Answer from the drawing. Dimensions are ordinates in mm from the lowest x, y and z of the part. Give positions to 0.01 mm unless a question says otherwise; leave off trailing zeros. Order: outer loops, then holes, each group sorted by start corner. A loop starts at its lowest first (then second) coordinate and runs counter-clockwise, first axis right, second up. Notation, with made-up numbers: (-28, 17) - (7, 17) arc R28 cw to (7, 50) - close; hole circle Ø7 at (83.25, -30.5). An arc over 180 degrees is marked (long way). Write each question's results on one line, items separated by ' | '.
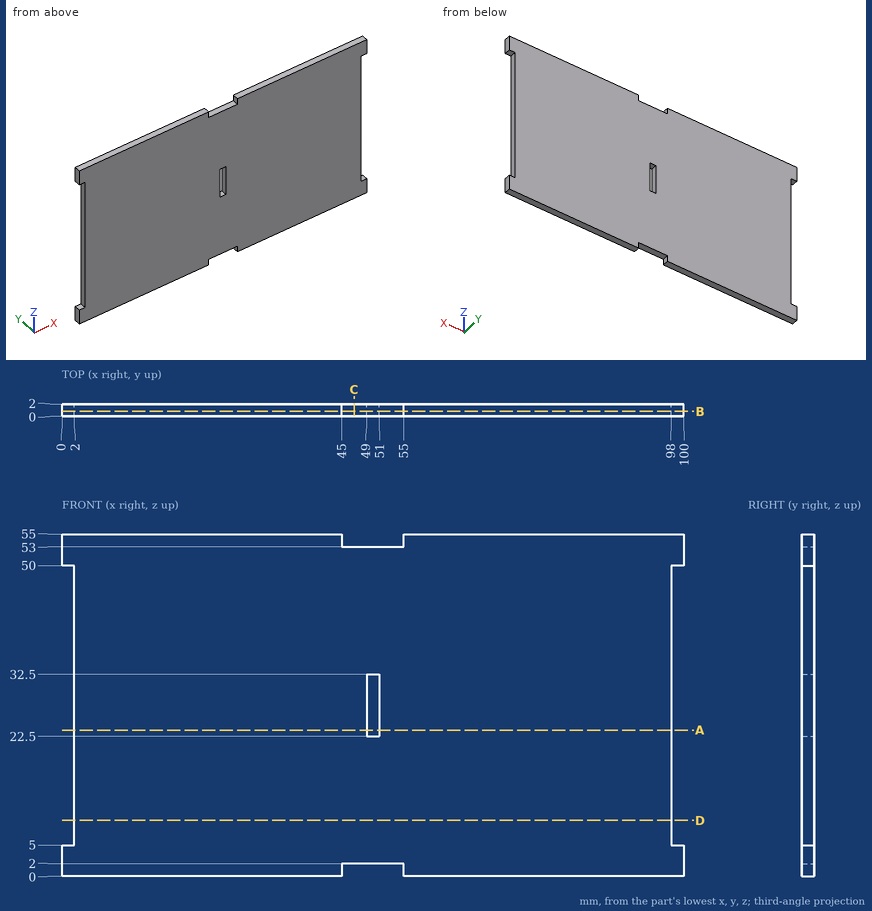
1. Given P1, Ø1, axis at y = 2, z = 23, coming from the +X side, flat-ended and moving along its own axis, determine where the tip first touches the part or whether it passes through.
Answer list:
P1: x = 98
2. A cutting plane is placed at B-B, the plane y = 0.8. Write down the section's boundary in (x, z), then the cut area to 3 significant figures.
Answer list:
outline: (0, 0) - (45, 0) - (45, 2) - (55, 2) - (55, 0) - (100, 0) - (100, 5) - (98, 5) - (98, 50) - (100, 50) - (100, 55) - (55, 55) - (55, 53) - (45, 53) - (45, 55) - (0, 55) - (0, 50) - (2, 50) - (2, 5) - (0, 5) - close; hole (49, 22.5) - (51, 22.5) - (51, 32.5) - (49, 32.5) - close | area: 5,260 mm^2
3. Straight lines are drawn through the part: line 1 (X direction, y = 0.5, z = 31); line 2 (X direction, y = 1, z = 43). For each, find the intervals that lie inside material, in ascending order. Write a range as [from, to].
Answer list:
line 1: [2, 49], [51, 98] | line 2: [2, 98]
4. A cutting plane is placed at D-D, the plane z = 9. Write down the section's boundary in (x, y).
Answer list:
outline: (2, 0) - (98, 0) - (98, 2) - (2, 2) - close
5. A cutting plane is placed at A-A, the plane z = 23.5. Write down the section's boundary in (x, y).
Answer list:
outline: (2, 0) - (49, 0) - (49, 2) - (2, 2) - close; (51, 0) - (98, 0) - (98, 2) - (51, 2) - close
6. A cutting plane is placed at C-C, the plane x = 47. Write down the section's boundary in (y, z), then the cut area to 3 significant figures.
Answer list:
outline: (0, 2) - (2, 2) - (2, 53) - (0, 53) - close | area: 102 mm^2
